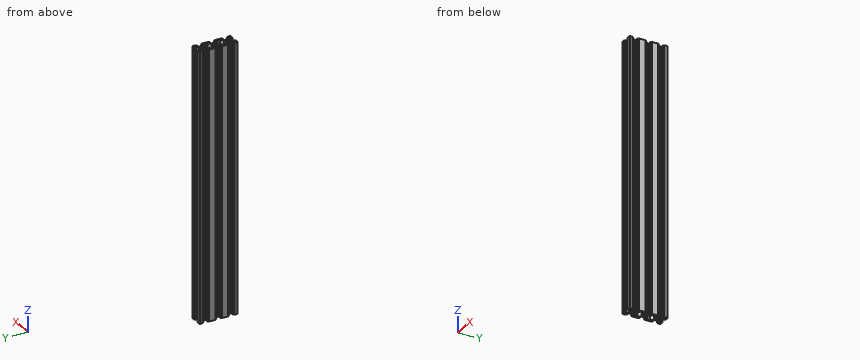
```python
from build123d import *

# Parameters (mm, degrees)
F0_R     = 2.1
F1_DEPTH = 421


with BuildPart() as f1:
    # F0 (on Top) → F1 (new body)
    with BuildSketch(Plane.XY):
        with BuildLine():
            Line((-8, -3), (-10, -5))
            Line((-10, -5), (-10, -15))
            Line((-10, -15), (-8, -17))
            Line((-8, -17), (-8, -14))
            Line((-8, -14), (-7.06066, -14))
            Line((-7.06066, -14), (-4, -17.06066))
            Line((-4, -17.06066), (-4, -19.480385))
            Line((-4, -19.480385), (-3.7, -20))
            Line((-3.7, -20), (-4, -20.519615))
            Line((-4, -20.519615), (-4, -22.93934))
            Line((-4, -22.93934), (-7.06066, -26))
            Line((-7.06066, -26), (-8, -26))
            Line((-8, -26), (-8, -23))
            Line((-8, -23), (-10, -25))
            Line((-10, -25), (-10, -29))
            ThreePointArc((-10, -29), (-9.707107, -29.707107), (-9, -30))
            Line((-9, -30), (-5, -30))
            Line((-5, -30), (-3, -28))
            Line((-3, -28), (-6, -28))
            Line((-6, -28), (-6, -27.06066))
            Line((-6, -27.06066), (-2.93934, -24))
            Line((-2.93934, -24), (-0.519615, -24))
            Line((-0.519615, -24), (0, -23.7))
            Line((0, -23.7), (0.519615, -24))
            Line((0.519615, -24), (2.93934, -24))
            Line((2.93934, -24), (6, -27.06066))
            Line((6, -27.06066), (6, -28))
            Line((6, -28), (3, -28))
            Line((3, -28), (5, -30))
            Line((5, -30), (9, -30))
            ThreePointArc((9, -30), (9.707107, -29.707107), (10, -29))
            Line((10, -29), (10, -25))
            Line((10, -25), (8, -23))
            Line((8, -23), (8, -26))
            Line((8, -26), (7.06066, -26))
            Line((7.06066, -26), (4, -22.93934))
            Line((4, -22.93934), (4, -20.519615))
            Line((4, -20.519615), (3.7, -20))
            Line((3.7, -20), (4, -19.480385))
            Line((4, -19.480385), (4, -17.06066))
            Line((4, -17.06066), (7.06066, -14))
            Line((7.06066, -14), (8, -14))
            Line((8, -14), (8, -17))
            Line((8, -17), (10, -15))
            Line((10, -15), (10, -5))
            Line((10, -5), (8, -3))
            Line((8, -3), (8, -6))
            Line((8, -6), (7.06066, -6))
            Line((7.06066, -6), (4, -2.93934))
            Line((4, -2.93934), (4, -0.519615))
            Line((4, -0.519615), (3.7, 0))
            Line((3.7, 0), (4, 0.519615))
            Line((4, 0.519615), (4, 2.93934))
            Line((4, 2.93934), (7.06066, 6))
            Line((7.06066, 6), (8, 6))
            Line((8, 6), (8, 3))
            Line((8, 3), (10, 5))
            Line((10, 5), (10, 15))
            Line((10, 15), (8, 17))
            Line((8, 17), (8, 14))
            Line((8, 14), (7.06066, 14))
            Line((7.06066, 14), (4, 17.06066))
            Line((4, 17.06066), (4, 19.480385))
            Line((4, 19.480385), (3.7, 20))
            Line((3.7, 20), (4, 20.519615))
            Line((4, 20.519615), (4, 22.93934))
            Line((4, 22.93934), (7.06066, 26))
            Line((7.06066, 26), (8, 26))
            Line((8, 26), (8, 23))
            Line((8, 23), (10, 25))
            Line((10, 25), (10, 29))
            ThreePointArc((10, 29), (9.707107, 29.707107), (9, 30))
            Line((9, 30), (5, 30))
            Line((5, 30), (3, 28))
            Line((3, 28), (6, 28))
            Line((6, 28), (6, 27.06066))
            Line((6, 27.06066), (2.93934, 24))
            Line((2.93934, 24), (0.519615, 24))
            Line((0.519615, 24), (0, 23.7))
            Line((0, 23.7), (-0.519615, 24))
            Line((-0.519615, 24), (-2.93934, 24))
            Line((-2.93934, 24), (-6, 27.06066))
            Line((-6, 27.06066), (-6, 28))
            Line((-6, 28), (-3, 28))
            Line((-3, 28), (-5, 30))
            Line((-5, 30), (-9, 30))
            ThreePointArc((-9, 30), (-9.707107, 29.707107), (-10, 29))
            Line((-10, 29), (-10, 25))
            Line((-10, 25), (-8, 23))
            Line((-8, 23), (-8, 26))
            Line((-8, 26), (-7.06066, 26))
            Line((-7.06066, 26), (-4, 22.93934))
            Line((-4, 22.93934), (-4, 20.519615))
            Line((-4, 20.519615), (-3.7, 20))
            Line((-3.7, 20), (-4, 19.480385))
            Line((-4, 19.480385), (-4, 17.06066))
            Line((-4, 17.06066), (-7.06066, 14))
            Line((-7.06066, 14), (-8, 14))
            Line((-8, 14), (-8, 17))
            Line((-8, 17), (-10, 15))
            Line((-10, 15), (-10, 5))
            Line((-10, 5), (-8, 3))
            Line((-8, 3), (-8, 6))
            Line((-8, 6), (-7.06066, 6))
            Line((-7.06066, 6), (-4, 2.93934))
            Line((-4, 2.93934), (-4, 0.519615))
            Line((-4, 0.519615), (-3.7, 0))
            Line((-3.7, 0), (-4, -0.519615))
            Line((-4, -0.519615), (-4, -2.93934))
            Line((-4, -2.93934), (-7.06066, -6))
            Line((-7.06066, -6), (-8, -6))
            Line((-8, -6), (-8, -3))
        make_face()
        with Locations((0, -20)):
            Circle(F0_R, mode=Mode.SUBTRACT)
        Polygon((-8, -8), (-6.93934, -8), (-2.93934, -4), (2.93934, -4), (6.93934, -8), (8, -8), (8, -12), (6.93934, -12), (2.93934, -16), (-2.93934, -16), (-6.93934, -12), (-8, -12), align=None, mode=Mode.SUBTRACT)
        Circle(F0_R, mode=Mode.SUBTRACT)
        Polygon((-8, 8), (-8, 12), (-6.93934, 12), (-2.93934, 16), (2.93934, 16), (6.93934, 12), (8, 12), (8, 8), (6.93934, 8), (2.93934, 4), (-2.93934, 4), (-6.93934, 8), align=None, mode=Mode.SUBTRACT)
        with Locations((0, 20)):
            Circle(F0_R, mode=Mode.SUBTRACT)
    extrude(amount=F1_DEPTH)


solid = f1.part
```
Here's how the part is built. I have some questions about the finished solid (model axes, mm). Give positions to 0.01 mm unless a question says otherwise; leave off trailing zeros.
(1) Will these pins go through, and if not, where does the flat tip stop? pin 1 (2 mm diameter, centred on x = 0.5, z = 140, fed in from -Y); pin 2 (4.5 mm diameter, centred on x = 0, z = 116, fed in from +Y); pin 3 (2 mm diameter, centred on y = -15.5, z = 116, fed in from -X); pin 4 (6 mm diameter, centred on y = -21.5, z = 138, fed in from +X).
Output values:
pin 1: stops at y = -24
pin 2: stops at y = 24
pin 3: stops at x = -10
pin 4: stops at x = 9.5
(2) Imagine slicing it at A-A, the plane z = 306.5. Count the separate pieces of the cut face and the enclosed holes in it, and give its area (3 significant figures).
Output values:
separate pieces: 1
enclosed holes: 5
area: 433 mm2
(3) If I drill on L1, parallel to Y at x = 0, z = 155.5; L2, parallel to Y at x = -7.5, z = 306; L3, parallel to X at y = -25, z = 329.5, over which ranges is the centre line in solid material (lowest first)?
Output values:
L1: y = -23.7 to -22.1, -17.9 to -16, -4 to -2.1, 2.1 to 4, 16 to 17.9, 22.1 to 23.7
L2: y = -30 to -26, -14 to -12, -8 to -6, 6 to 8, 12 to 14, 26 to 30
L3: x = -10 to -8, -6.06 to -3.94, 3.94 to 6.06, 8 to 10
